Source: CAD feature listing. Evaluate the final solid. Frame: model axes, mm. Round coordinates to 2 decimals unless told otherwise and drop trailing zeros. Write each loop counter-clockwise with the first axis right and the second up, starting at its lowest first coordinate (ties: lowest second). Pieces come first, ordered by that corner, then holes.
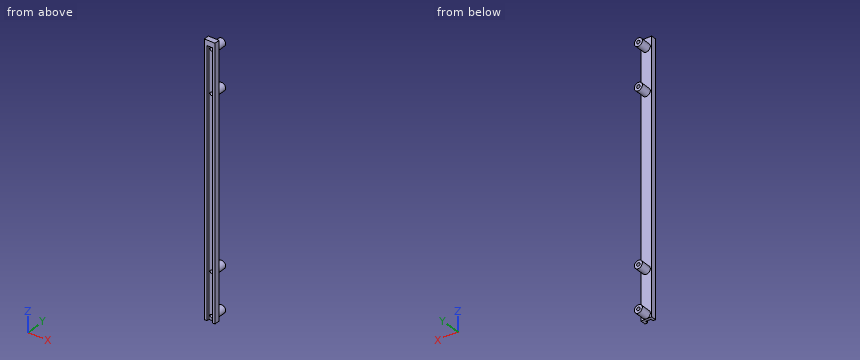
Autodesk Inventor part; units mm, degrees
ref_plane "YZ Plane" through (0, 0, 0) normal (1, 0, 0) x (0, 1, 0)
ref_plane "XZ Plane" through (0, 0, 0) normal (0, 1, 0) x (-1, 0, 0)
ref_plane "XY Plane" through (0, 0, 0) normal (0, 0, 1) x (1, 0, 0)
sketch "Sketch1" plane through (0, 0, 0) normal (0, 0, 1) x (1, 0, 0)
  line L0 (3.175, 0) -> (3.175, 3.175)
  line L1 (3.175, 3.175) -> (-3.175, 3.175)
  line L2 (-3.175, 3.175) -> (-3.175, 0)
  line L3 (6.35, 0) -> (6.35, 6.35)
  line L4 (6.35, 6.35) -> (-6.35, 6.35)
  line L5 (-6.35, 6.35) -> (-6.35, 0)
  line L6 (-6.35, 0) -> (-3.175, 0)
  line L7 (3.175, 0) -> (6.35, 0)
  point P0 (0, 0)
extrude "Extrusion1" add sketch "Sketch1" along normal blind 314.325
sketch "Sketch2" plane through (-6.35, 6.35, 0) normal (0, 1, 0) x (1, 0, 0)
  circle A0 centre (6.35, -4.7625) radius 1.985
  circle A1 centre (6.35, -55.5625) radius 1.985
  circle A2 centre (6.35, -309.5625) radius 1.985
  circle A3 centre (6.35, -258.7625) radius 1.985
  point P0 (6.35, 0)
  dimension "d2" = 3.97
  dimension "d3" = 3.97
  dimension "d4" = 3.97
  dimension "d5" = 3.97
extrude "Extrusion2" cut sketch "Sketch2" against normal blind 314.325
sketch "Sketch3" plane through (-6.35, 6.35, 0) normal (0, 1, 0) x (1, 0, 0)
  circle A0 centre (6.35, -4.7625) radius 1.985
  circle A1 centre (6.35, -55.5625) radius 1.985
  circle A2 centre (6.35, -258.7625) radius 1.985
  circle A3 centre (6.35, -309.5625) radius 1.985
  circle A4 centre (6.35, -4.7625) radius 4.7625
  circle A5 centre (6.35, -55.5625) radius 4.7625
  circle A6 centre (6.35, -258.7625) radius 4.7625
  circle A7 centre (6.35, -309.5625) radius 4.7625
  point P0 (6.35, 0)
extrude "Extrusion3" add sketch "Sketch3" along normal blind 12.7
sketch "Sketch4" plane through (0, 0, 314.325) normal (0, 0, 1) x (1, 0, 0)
  line L0 (-6.35, 0) -> (-3.175, 0)
  line L1 (-6.35, 0) -> (6.35, 0)
  line L2 (6.35, 0) -> (6.35, 6.35)
  line L3 (6.35, 6.35) -> (-6.35, 6.35)
  line L4 (-6.35, 6.35) -> (-6.35, 0)
  point P0 (0, 0)
extrude "Extrusion4" add sketch "Sketch4" along normal blind 6.35
properties part number "crossbrace_jig"
1) Section query A-A on y = 11. Return the cut outline in (x, z) (1 decimal), then the cut area to 3 significant figures.
Taken from the geometry:
outline: circle Ø9.5 at (0, 4.8); circle Ø9.5 at (0, 55.6); circle Ø9.5 at (0, 258.8); circle Ø9.5 at (0, 309.6); hole circle Ø4 at (0, 4.8); hole circle Ø4 at (0, 55.6); hole circle Ø4 at (0, 258.8); hole circle Ø4 at (0, 309.6)
area: 236 mm2
2) Contact query for flat-ended pins moving along their axis: P1, Ø1.6, axis at x = 1.5, y = 1.5, coming from the -Z side (3 decimals); P2, Ø4, axis at x = 2.5, y = 14, coming from the +Z side; P3, Ø4, axis at y = 13.5, z = 54, coming from the -X side; P4, Ø2.5, axis at x = 0, z = 309.56, coming from the +Y side. Output: stop coordinate, or through.
Taken from the geometry:
P1: stops at z = 314.325
P2: stops at z = 314.3
P3: stops at x = -4.76
P4: passes through
3) Section query B-B on z = 269. Return the cut outline in (x, y) (3 decimals).
Taken from the geometry:
outline: (-6.35, 0) - (-3.175, 0) - (-3.175, 3.175) - (3.175, 3.175) - (3.175, 0) - (6.35, 0) - (6.35, 6.35) - (-6.35, 6.35) - close
4) Material intervals for line 1 (Z direction, x = 0, y = 5.75) (1 decimal); line 2 (Z direction, x = -2.75, y = 12.5); line 3 (Z direction, x = -0.75, y = 3.5) (3 decimals), sorted ascending.
Taken from the geometry:
line 1: z = 0 to 2.8, 6.7 to 53.6, 57.5 to 256.8, 260.7 to 307.6, 311.5 to 320.7
line 2: z = 0.87 to 8.65, 51.67 to 59.45, 254.87 to 262.65, 305.67 to 313.45
line 3: z = 0 to 2.925, 6.6 to 53.725, 57.4 to 256.925, 260.6 to 307.725, 311.4 to 320.675
